Could you check a few things on this model? Use its own coordinates, in mm. A direction names the side the tool comes from. Coordinates: 2 decimals unless noted, no trailing zeros. Loops run counter-clockwise (first coordinate to the right, second up) from the corner with the lowest first, then second, coordinate; pieces in that order, holes last.
from build123d import *

# Parameters (mm, degrees)
SKETCH_1_R               = 10.25
EXTRUDE_1_DEPTH          = 2.2
SKETCH_2_R               = 3.85
SKETCH_2_R_2             = 2.6
EXTRUDE_2_DEPTH          = 3.1
SKETCH_3_R               = 0.75
SKETCH_3_R_2             = 1.5
CUT_EXTRUDE_1_DEPTH      = 3.2
SKETCH_4_R               = 4.25
SKETCH_4_R_2             = 3.25
SKETCH_4_R_3             = 3
SKETCH_4_R_4             = 1.5
CUT_EXTRUDE_2_DEPTH      = 1
SKETCH_5_R               = 2.6
SKETCH_5_R_2             = 1.5
EXTRUDE_3_DEPTH          = 0.3
CUT_EXTRUDE_3_DEPTH      = 2.8
PATTERN_CIRCULAR_1_COUNT = 26


with BuildPart() as part:
    # Эскиз1 → Бобышка-Вытянуть1 (new body)
    with BuildSketch(Plane(origin=(0, 0, 0), x_dir=(1, 0, 0), z_dir=(0, 1, 0))):
        Circle(SKETCH_1_R)
    extrude(amount=EXTRUDE_1_DEPTH)

    # Эскиз2 → Бобышка-Вытянуть2 (add)
    with BuildSketch(Plane(origin=(0, 2.2, 0), x_dir=(1, 0, 0), z_dir=(0, 1, 0))):
        Circle(SKETCH_2_R)
        Circle(SKETCH_2_R_2, mode=Mode.SUBTRACT)
    extrude(amount=EXTRUDE_2_DEPTH)

    # Эскиз3 → Вырез-Вытянуть1 (cut, through all)
    with BuildSketch(Plane(origin=(0, 2.2, 0), x_dir=(1, 0, 0), z_dir=(0, 1, 0))):
        with Locations((0, 7.2)):
            Circle(SKETCH_3_R)
        with Locations((7.2, 0)):
            Circle(SKETCH_3_R)
        with Locations((0, -7.2)):
            Circle(SKETCH_3_R)
        with Locations((-7.2, 0)):
            Circle(SKETCH_3_R)
        Circle(SKETCH_3_R_2)
        with Locations((2.75, 7.2)):
            Circle(SKETCH_3_R)
        with Locations((2.75, -7.2)):
            Circle(SKETCH_3_R)
        with Locations((-2.75, 7.2)):
            Circle(SKETCH_3_R)
        with Locations((-2.75, -7.2)):
            Circle(SKETCH_3_R)
        with Locations((7.2, 2.75)):
            Circle(SKETCH_3_R)
        with Locations((-7.2, 2.75)):
            Circle(SKETCH_3_R)
        with Locations((7.2, -2.75)):
            Circle(SKETCH_3_R)
        with Locations((-7.2, -2.75)):
            Circle(SKETCH_3_R)
    extrude(amount=-CUT_EXTRUDE_1_DEPTH, mode=Mode.SUBTRACT)

    # Эскиз4 → Вырез-Вытянуть2 (cut)
    with BuildSketch(Plane.XZ):
        Circle(SKETCH_4_R)
        Circle(SKETCH_4_R_2, mode=Mode.SUBTRACT)
        Circle(SKETCH_4_R_3)
        Circle(SKETCH_4_R_4, mode=Mode.SUBTRACT)
    extrude(amount=-CUT_EXTRUDE_2_DEPTH, mode=Mode.SUBTRACT)

    # Эскиз5 → Бобышка-Вытянуть3 (add)
    with BuildSketch(Plane(origin=(0, 2.2, 0), x_dir=(1, 0, 0), z_dir=(0, 1, 0))):
        Circle(SKETCH_5_R)
        Circle(SKETCH_5_R_2, mode=Mode.SUBTRACT)
    extrude(amount=EXTRUDE_3_DEPTH)

    # Эскиз6 → Вырез-Вытянуть3 (cut)
    with BuildSketch(Plane(origin=(0, 5.3, 0), x_dir=(1, 0, 0), z_dir=(0, 1, 0))):
        with BuildLine():
            Line((0, 2.9), (-0.262912611, 2.586672952))
            ThreePointArc((-0.262912611, 2.586672952), (0, 2.6), (0.262912611, 2.586672952))
            Line((0.262912611, 2.586672952), (0, 2.9))
        make_face()
    cut_extrude_3 = extrude(amount=-CUT_EXTRUDE_3_DEPTH, mode=Mode.SUBTRACT)

    # Круговой массив1: Вырез-Вытянуть3 ×26 about axis
    pattern_circular_1_axis = Axis((0, 0, 0), (0, 1, 0))
    for i in range(1, PATTERN_CIRCULAR_1_COUNT):
        add(cut_extrude_3.rotate(pattern_circular_1_axis, i * 360 / PATTERN_CIRCULAR_1_COUNT), mode=Mode.SUBTRACT)


solid = part.part
1) We'd pull the mould along Z, two halves only. Please class faces 1 (the cylindrical face through (-7.95, 1.12, -2.78)), 2 (the cylindrical face through (-2.222, 1.085, 10.006)), 3 (the flat face through (-1, 5.3, 3)), 4 (the cylindrical face through (6.45, 1.12, -0.03)): released by +Z, released by -Z, zero draft, split by the parting line, or undercut.
2) Imagine slicing it at D-D on z = -9. List the corners of the cut face in (x, y) for me.
3) Imagine slicing it at C-C on z = 8.25. List the corners of the cut face in (x, y) for me, plus the area to 3 significant figures.
4) Imagine slicing it at A-A on y = 1.35. State how many separate pieces and enclosed holes the cut face has, plus the area to 3 significant figures.
5) For faces 5 (the cylindrical face through (-0.83, 3.73, 3.76)), 6 (the flat face through (1.3, 1, -1.3)), 7 (the cylindrical face through (-2.848, 1.115, 6.456)), which set-ups out of +Z, -Z, +X, -X, +Y, -Y let a thin tool reach every point of the face, with its end or its side?
6) Imagine slicing it at B-B on x = -7.2. List the corners of the cut face in (y, z) for me.
7) Will these pins go through, and if not, where does the flat tip stop? pin 1 (2 mm diameter, centred on x = 2, y = 3.5, fed in from -Z); pin 2 (4 mm diameter, centred on x = 0, z = 0, fed in from +Y); pin 3 (3 mm diameter, centred on y = 2, z = 5.5, fed in from +X).
8) If I drill on L1, parallel to Z at x = 7.2, y = 1.65; L2, parallel to Z at x = 2.75, y = 1.5; L3, parallel to X at y = 0.25, z = 7.75, over which ranges is the centre line in solid material (lowest first)?
Solved:
1. face 1: undercut
1. face 2: split by the parting line
1. face 3: zero draft
1. face 4: undercut
2. outline: (-4.91, 0) - (4.91, 0) - (4.91, 2.2) - (-4.91, 2.2) - close
3. outline: (-6.08, 0) - (6.08, 0) - (6.08, 2.2) - (-6.08, 2.2) - close
3. area: 26.8 mm2
4. separate pieces: 1
4. enclosed holes: 13
4. area: 302 mm2
5. face 5: +Y
5. face 6: -Y
5. face 7: +Y, -Y
6. outline: (0, -7.3) - (2.2, -7.3) - (2.2, -3.5) - (0, -3.5) - close; (0, -2) - (2.2, -2) - (2.2, -0.75) - (0, -0.75) - close; (0, 0.75) - (2.2, 0.75) - (2.2, 2) - (0, 2) - close; (0, 3.5) - (2.2, 3.5) - (2.2, 7.3) - (0, 7.3) - close
7. pin 1: stops at z = -3.72
7. pin 2: stops at y = 2.5
7. pin 3: stops at x = 9.44
8. L1: z = -7.3 to -3.5, -2 to -0.75, 0.75 to 2, 3.5 to 7.3
8. L2: z = -9.87 to -7.95, -6.45 to 6.45, 7.95 to 9.87
8. L3: x = -6.71 to -3.26, -2.24 to -0.51, 0.51 to 2.24, 3.26 to 6.71
